Verification items for the finished model (mm, model axes). Coordinates: 2 decimals unless noted, no trailing zeros. Order: outer loops, then holes, each group sorted by start corner. A loop starts at its lowest first (then second) coordinate and runs counter-clockwise, first axis right, second up.
Q1. Cross-section at D-D, the plane x = 34. Record the boundary of the cut face in (y, z), and give its area (3 significant figures).
Q2. Cross-section at C-C, the plane y = -1.25. Record the boundary of the cut face in (x, z), and give its area (3 significant figures).
Q3. Cross-section at B-B, the plane x = 0. Record the boundary of the cut face in (y, z), and give its area (3 significant figures).
Q4. Depth check by flat-ended pin: P1, Ø2, axis at x = -9, y = 1.5, coming from the +Z side; P2, Ø1, axis at y = 0, z = 6.5, coming from the -X side; P3, Ø5, axis at x = 24.5, y = -2, coming from the -Z side; P4, Ø3, axis at x = 25, z = -10.5, coming from the +Y side. Enter the tip coordinate at first touch or a pass-through.
Q5. Cross-section at A-A, the plane z = 0. Record the boundary of the cut face in (x, y).
Q6. Thickness scan on line 1 (X direction, y = 1.2, z = 0); line 2 (Y direction, x = -1, z = -7); line 3 (Z direction, x = 8, y = 1). Record the ranges inside material, lowest first.
from build123d import *

# Parameters (mm, degrees)
SKETCH_1_R      = 1.5
SKETCH_1_R_2    = 2
EXTRUDE_1_DEPTH = 2
SKETCH_2_W      = 10
SKETCH_2_H      = 2
EXTRUDE_2_DEPTH = 10
FILLET_1_R      = 3
FILLET_2_R      = 3


with BuildPart() as part:
    # 草图1 → 凸台-拉伸1 (new body)
    with BuildSketch(Plane(origin=(0, 0, 0), x_dir=(1, 0, 0), z_dir=(0, 1, 0))):
        with BuildLine():
            Line((-32, 5), (0, 17))
            Line((0, 17), (40, 5))
            Line((40, 5), (40, -5))
            Line((40, -5), (-32, -5))
            ThreePointArc((-32, -5), (-37, 0), (-32, 5))
        make_face()
        with Locations(Location((-32, 0, 0), (0, 0, 270))):
            Circle(SKETCH_1_R, mode=Mode.SUBTRACT)
        with Locations(Location((0, 0, 0), (0, 0, 270))):
            Circle(SKETCH_1_R_2, mode=Mode.SUBTRACT)
    extrude(amount=EXTRUDE_1_DEPTH)

    # 草图2 → 凸台-拉伸2 (add)
    with BuildSketch(Plane(origin=(0, 2, 0), x_dir=(1, 0, 0), z_dir=(0, 1, 0))):
        with Locations((35, -6)):
            Rectangle(SKETCH_2_W, SKETCH_2_H)
    extrude(amount=-EXTRUDE_2_DEPTH)

    # 圆角1
    fillet_1_edges = [part.edges().sort_by_distance(p)[0] for p in [
        (-32, 1, -5),
        (0, 1, -17),
        (40, 1, -5),
    ]]
    fillet(fillet_1_edges, radius=FILLET_1_R)

    # 圆角2
    fillet_2_edges = [part.edges().sort_by_distance(p)[0] for p in [
        (40, -8, 6),
        (30, -8, 6),
    ]]
    fillet(fillet_2_edges, radius=FILLET_2_R)


solid = part.part
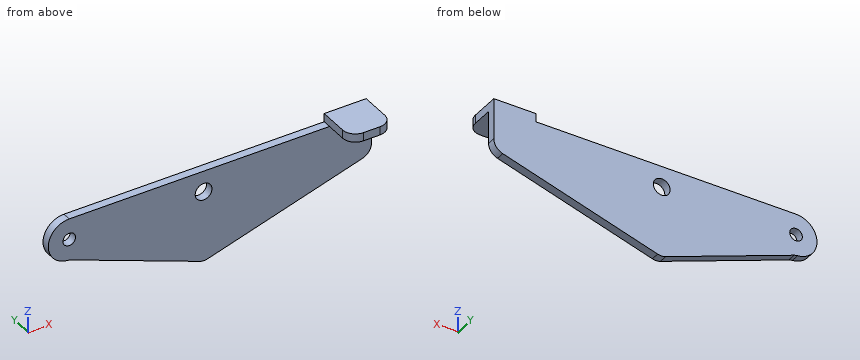
Check values:
1. outline: (-8, 5) - (0, 5) - (0, -6.8) - (2, -6.8) - (2, 7) - (-8, 7) - close
1. area: 43.6 mm2
2. outline: (30, 5) - (40, 5) - (40, 7) - (30, 7) - close
2. area: 20.0 mm2
3. outline: (0, -16.83) - (2, -16.83) - (2, -2) - (0, -2) - close; (0, 2) - (2, 2) - (2, 5) - (0, 5) - close
3. area: 35.7 mm2
4. P1: stops at z = 5
4. P2: stops at x = 30
4. P3: stops at z = -10.1
4. P4: stops at y = 2
5. outline: (-37, 0) - (-33.5, 0) - (-33.5, 2) - (-37, 2) - close; (-30.5, 0) - (-2, 0) - (-2, 2) - (-30.5, 2) - close; (2, 0) - (40, 0) - (40, 2) - (2, 2) - close
6. line 1: x = -37 to -33.5, -30.5 to -2, 2 to 40
6. line 2: y = 0 to 2
6. line 3: z = -14.6 to 5
